Verification items for the finished model (mm, model axes). A direction names the side the tool comes from. Coordinates: 2 decimals unless noted, no trailing zeros. Loops run counter-clockwise (first coordinate to the right, second up) from the corner with the lowest first, then second, coordinate; pieces in that order, holes last. Notation, with made-up numbers: (49, -6.75) -> (107, -6.75) arc R24 ccw to (107, 14.25) -> close; hole circle Ø3 at (72.25, 87.25). An arc over 180 degrees is marked (long way). Use CSV: the item, a comma, the result in double quotes. Start each with the question number.
```python
from build123d import *

# Parameters (mm, degrees)
F0_W      = 27
F0_H      = 15.9
F0_W_2    = 15.9
F0_H_2    = 27
F0_W_3    = 3
F0_H_3    = 3
F1_DEPTH  = 21.9
F2_DEPTH  = 51.8
F3_R      = 7.95
F6_DEPTH  = 30
F7_DEPTH  = 30
F4_R      = 7.9
F8_DEPTH  = 30
F10_DEPTH = 58.2
F11_W     = 3
F11_H     = 13.3
F13_R     = 1.5


with BuildPart() as f1:
    # F0 (on Front) → F1 (new body)
    with BuildSketch(Plane.XZ):
        with BuildLine():
            Line((-34.3576915575, 15.9), (-42.3076915575, 15.9))
            Line((-42.3076915575, 15.9), (-42.3076915575, 7.9499999931))
            ThreePointArc((-42.3076915575, 7.9499999931), (-39.9791904704, 13.571498908), (-34.3576915575, 15.9))
        make_face()
        with BuildLine():
            ThreePointArc((-34.3576915575, 15.9), (-39.9791904704, 13.571498908), (-42.3076915575, 7.9499999931))
            ThreePointArc((-42.3076915575, 7.9499999931), (-39.9791904655, 2.3285010871), (-34.3576915575, 0))
            ThreePointArc((-34.3576915575, 0), (-28.7361926471, 2.3285010896), (-26.4076915575, 7.95))
            ThreePointArc((-26.4076915575, 7.95), (-28.7361926471, 13.5714989104), (-34.3576915575, 15.9))
        make_face()
        Polygon((-42.3076915575, 18.9), (-42.3076915575, 45.9), (-26.4076915575, 45.9), (-26.4076915575, 18.9), (-23.4076915575, 18.9), (-23.4076915575, 48.9), (-45.3076915575, 48.9), (-45.3076915575, 18.9), align=None)
        with Locations((-9.9076915575, 7.95)):
            Rectangle(F0_W, F0_H)
        with Locations((-34.3576915575, 32.4)):
            Rectangle(F0_W_2, F0_H_2)
        with BuildLine():
            ThreePointArc((-34.3576915575, 0), (-39.9791904655, 2.3285010871), (-42.3076915575, 7.9499999931))
            Line((-42.3076915575, 7.9499999931), (-42.3076915575, 0))
            Line((-42.3076915575, 0), (-34.3576915575, 0))
        make_face()
        with BuildLine():
            Line((-26.4076915575, 0), (-26.4076915575, 7.95))
            ThreePointArc((-26.4076915575, 7.95), (-28.7361926471, 2.3285010896), (-34.3576915575, 0))
            Line((-34.3576915575, 0), (-26.4076915575, 0))
        make_face()
        with BuildLine():
            Line((-26.4076915575, 7.95), (-26.4076915575, 15.9))
            Line((-26.4076915575, 15.9), (-34.3576915575, 15.9))
            ThreePointArc((-34.3576915575, 15.9), (-28.7361926471, 13.5714989104), (-26.4076915575, 7.95))
        make_face()
        Polygon((6.5923084425, 18.9), (-23.4076915575, 18.9), (-23.4076915575, 15.9), (3.5923084425, 15.9), (3.5923084425, 0), (-23.4076915575, 0), (-23.4076915575, -3), (6.5923084425, -3), align=None)
        Polygon((-26.4076915575, 18.9), (-42.3076915575, 18.9), (-42.3076915575, 15.9), (-34.3576915575, 15.9), (-26.4076915575, 15.9), align=None)
        Polygon((-23.4076915575, 15.9), (-26.4076915575, 15.9), (-26.4076915575, 7.95), (-26.4076915575, 0), (-23.4076915575, 0), align=None)
        Polygon((-42.3076915575, 15.9), (-42.3076915575, 18.9), (-45.3076915575, 18.9), (-45.3076915575, -3), (-23.4076915575, -3), (-23.4076915575, 0), (-26.4076915575, 0), (-34.3576915575, 0), (-42.3076915575, 0), (-42.3076915575, 7.9499999931), align=None)
        with Locations((-24.9076915575, 17.4)):
            Rectangle(F0_W_3, F0_H_3)
    extrude(amount=F1_DEPTH)

    # F0 (on Front) → F2 (join)
    with BuildSketch(Plane.XZ):
        Polygon((-42.3076915575, 15.9), (-42.3076915575, 18.9), (-45.3076915575, 18.9), (-45.3076915575, -3), (-23.4076915575, -3), (-23.4076915575, 0), (-26.4076915575, 0), (-34.3576915575, 0), (-42.3076915575, 0), (-42.3076915575, 7.9499999931), align=None)
        with BuildLine():
            ThreePointArc((-34.3576915575, 15.9), (-39.9791904704, 13.571498908), (-42.3076915575, 7.9499999931))
            ThreePointArc((-42.3076915575, 7.9499999931), (-39.9791904655, 2.3285010871), (-34.3576915575, 0))
            ThreePointArc((-34.3576915575, 0), (-28.7361926471, 2.3285010896), (-26.4076915575, 7.95))
            ThreePointArc((-26.4076915575, 7.95), (-28.7361926471, 13.5714989104), (-34.3576915575, 15.9))
        make_face()
        Polygon((-26.4076915575, 18.9), (-42.3076915575, 18.9), (-42.3076915575, 15.9), (-34.3576915575, 15.9), (-26.4076915575, 15.9), align=None)
        Polygon((-23.4076915575, 15.9), (-26.4076915575, 15.9), (-26.4076915575, 7.95), (-26.4076915575, 0), (-23.4076915575, 0), align=None)
        with Locations((-24.9076915575, 17.4)):
            Rectangle(F0_W_3, F0_H_3)
        with BuildLine():
            Line((-26.4076915575, 7.95), (-26.4076915575, 15.9))
            Line((-26.4076915575, 15.9), (-34.3576915575, 15.9))
            ThreePointArc((-34.3576915575, 15.9), (-28.7361926471, 13.5714989104), (-26.4076915575, 7.95))
        make_face()
        with BuildLine():
            Line((-34.3576915575, 15.9), (-42.3076915575, 15.9))
            Line((-42.3076915575, 15.9), (-42.3076915575, 7.9499999931))
            ThreePointArc((-42.3076915575, 7.9499999931), (-39.9791904704, 13.571498908), (-34.3576915575, 15.9))
        make_face()
        with BuildLine():
            ThreePointArc((-34.3576915575, 0), (-39.9791904655, 2.3285010871), (-42.3076915575, 7.9499999931))
            Line((-42.3076915575, 7.9499999931), (-42.3076915575, 0))
            Line((-42.3076915575, 0), (-34.3576915575, 0))
        make_face()
        with BuildLine():
            Line((-26.4076915575, 0), (-26.4076915575, 7.95))
            ThreePointArc((-26.4076915575, 7.95), (-28.7361926471, 2.3285010896), (-34.3576915575, 0))
            Line((-34.3576915575, 0), (-26.4076915575, 0))
        make_face()
    extrude(amount=F2_DEPTH)

    # F3 (on face) → F6 (cut)
    with BuildSketch(Plane.XZ.offset(51.8)):
        with Locations((-34.3576915575, 7.95)):
            Circle(F3_R)
    extrude(amount=-F6_DEPTH, mode=Mode.SUBTRACT)

    # F5 (on face) → F7 (cut)
    with BuildSketch(Plane.YZ.offset(6.5923084425)):
        with BuildLine():
            ThreePointArc((-3, 7.95), (-5.3285010896, 13.5714989104), (-10.95, 15.9))
            ThreePointArc((-10.95, 15.9), (-16.5714989104, 13.5714989104), (-18.9, 7.95))
            ThreePointArc((-18.9, 7.95), (-16.5714989104, 2.3285010896), (-10.95, 0))
            ThreePointArc((-10.95, 0), (-5.3285010896, 2.3285010896), (-3, 7.95))
        make_face()
    extrude(amount=-F7_DEPTH, mode=Mode.SUBTRACT)

    # F4 (on face) → F8 (cut)
    with BuildSketch(Plane.XY.offset(48.9)):
        with Locations((-34.3576915575, -10.9)):
            Circle(F4_R)
    extrude(amount=-F8_DEPTH, mode=Mode.SUBTRACT)

    # F9 (on face) → F10 (join)
    with BuildSketch(Plane.XZ.offset(51.8)):
        Polygon((-51.6076915575, -3), (-45.3076915575, -3), (-45.3076915575, 0), (-48.6076915575, 0), (-48.6076915575, 13.3), (-51.6076915575, 13.3), align=None)
    extrude(amount=-F10_DEPTH)

    # F11 (on face) → F12 (join, up to the next surface of F1)
    with BuildSketch(Plane.YZ.offset(6.5923084425)):
        Polygon((6.4, -3), (6.4, 0), (3.4, 0), (0, 0), (0, -3), align=None)
        with Locations((4.9, 6.65)):
            Rectangle(F11_W, F11_H)
    extrude(until=Until.NEXT, dir=(-1, 0, 0))

    # F13
    f13_edges = [f1.edges().sort_by_distance(p)[0] for p in [
        (6.592308, 3.4, 6.65),
        (-48.607692, -51.8, 6.65),
    ]]
    fillet(f13_edges, radius=F13_R)


solid = f1.part
```
1. Set-up check for faces 1 (the cylindrical face through (-49.059, -51.372, 6.743)), 2 (the flat face through (-47, -11, 0)), 3 (the flat face through (-34, -37, 18.9)), 4 (the cylindrical face through (6.141, 3.828, 6.743)): record each of +Z, -Z, +X, -X, +Y, -Y from which the full face is reachable in a straight line by a thin tool's end or side.
2. Release check for a two-part mould opening along Y. For faces 5 (the cylindrical face through (-27.01, -37.01, 4.91)), 6 (the flat face through (-41, -51.8, 3)), 7 (the flat face through (-25, 0, 19)) record: released by +Y, released by -Y, zero draft, split by the parting line, or undercut.
3. Scan lines: line 1 (X direction, y = -37, z = 7); line 2 (Y direction, x = -15.5, z = 8); line 3 (Y direction, x = -33, z = 46). Record each from-to range of solid material in increasing order.
4. Depth check by flat-ended pin: pin 1 (12.5 mm diameter, centred on y = -11, z = 9, fed in from +X); pin 2 (11 mm diameter, centred on x = -35, z = 37.5, fed in from -Y); pin 3 (17.5 mm diameter, centred on x = -36, y = -41.5, fed in from +Z). Enter the tip coordinate at first touch or a pass-through.
5. Cross-section at B-B, the plane z = 21.5. Record the boundary of the cut face in (x, y).
6. Cross-section at C-C, the plane z = 9. Record the boundary of the cut face in (x, y), plus the area to 3 significant figures.
7. Cross-section at A-A, the plane x = -9. Record the boundary of the cut face in (y, z).
8. Cross-section at D-D, the plane z = 15. Record the boundary of the cut face in (x, y), plus the area to 3 significant figures.
Solution:
1,face 1,"+Z, -Y"
1,face 2,"+Z"
1,face 3,"+Z, +X, -X, -Y"
1,face 4,"+Z, +X"
2,face 5,"zero draft"
2,face 6,"released by -Y"
2,face 7,"undercut"
3,line 1,"x = -51.61 to -48.61, -45.31 to -42.25, -26.46 to -23.41"
3,line 2,"y = -21.9 to -18.9, -3 to 0, 3.4 to 6.4"
3,line 3,"y = -21.9 to -18.68, -3.12 to 0"
4,pin 1,"stops at x = -23.41"
4,pin 2,"stops at y = -21.9"
4,pin 3,"stops at z = 18.9"
5,outline,"(-45.31, -21.9) -> (-23.41, -21.9) -> (-23.41, 0) -> (-45.31, 0) -> close; hole circle Ø15.8 at (-34.36, -10.9)"
6,outline,"(-51.61, -51.8) -> (-50.11, -51.8) arc R1.5 ccw to (-48.61, -50.3) -> (-48.61, 3.4) -> (5.09, 3.4) arc R1.5 ccw to (6.59, 4.9) -> (6.59, 6.4) -> (-51.61, 6.4) -> close; (-45.31, -51.8) -> (-42.24, -51.8) -> (-42.24, -21.8) -> (-26.48, -21.8) -> (-26.48, -51.8) -> (-23.41, -51.8) -> (-23.41, -21.9) -> (6.59, -21.9) -> (6.59, -18.83) -> (-23.41, -18.83) -> (-23.41, -3.07) -> (6.59, -3.07) -> (6.59, 0) -> (-45.31, 0) -> close"
6,area,"1,190 mm2"
7,outline,"(-21.9, -3) -> (6.4, -3) -> (6.4, 13.3) -> (3.4, 13.3) -> (3.4, 0) -> (0, 0) -> (0, 18.9) -> (-21.9, 18.9) -> close; hole circle Ø15.9 at (-10.95, 7.95)"
8,outline,"(-45.31, -51.8) -> (-38.03, -51.8) -> (-38.03, -21.8) -> (-30.68, -21.8) -> (-30.68, -51.8) -> (-23.41, -51.8) -> (-23.41, -21.9) -> (6.59, -21.9) -> (6.59, -14.62) -> (-23.41, -14.62) -> (-23.41, -7.28) -> (6.59, -7.28) -> (6.59, 0) -> (-45.31, 0) -> close"
8,area,"1,350 mm2"
